For this review, take the finished solid that the model builds, in its own axes (mm). A direction names the side the tool comes from. Give positions to 0.01 mm unless a question says otherwise; leave off trailing zeros. Write each loop counter-clockwise with the first axis right and the second up, starting at its lowest first coordinate (ties: lowest second). Pieces come first, ordered by that corner, then holes.
1) We need section A-A on x = 0. Give the boundary of the cut face in (y, z).
2) We need section D-D on y = 101.5. Give the boundary of the cut face in (x, z), and give its area (3 significant figures).
3) For P1, Ø4, axis at x = -1, z = -91.5, coming from the +Y side; P2, Ø10, axis at x = 2.5, z = -95, coming from the -Y side; P3, Ø2.5, axis at x = -1, y = 93, coming from the -Z side; P4, Ø2, axis at x = -10, y = 76, coming from the +Z side, all flat-tipped, find the tip position at first contact; note any pin that passes through.
4) Wall thickness on line 1 along Y through (x, z) = (0, -77); line 2 along X through (y, z) = (92, -79.25); line 3 along Y through (x, z) = (-0.5, -97.5): over which ranges is each line inside the solid? List them lowest first.
5) We need section B-B on z = -80. Give the boundary of the cut face in (x, y), and give its area (3 significant figures).
6) Machinability: for faces 1 (the face through (-14, 92, -96)), 2 (the face through (-3.755, 103.923, -82.14)), 3 (the face through (-3.654, 94.071, -91.126)), which of the approach directions +Z, -Z, +X, -X, +Y, -Y give a long, thin tool a straight path to every point of the face, cutting with its end or side? Answer none if there is none.
7) Draft analysis for pull direction X (two halves, no side actions). For faces 4 (the face through (-13, 92, -92)), 5 (the face through (0, 96.2, -91)), 6 (the face through (3.654, 89.929, -91.126)), 7 (the face through (0.2, 117.5, -96.1)), state which applies: pulls with the +X half, pulls with the -X half, needs draft (parallel to the pull), parting line crosses it, or undercut.
8) We need section C-C on x = 8.75. Give the boundary of the cut face in (y, z).
from build123d import *

# Parameters (mm, degrees)
SKETCH151_W     = 65
SKETCH151_H     = 65
SKETCH151_W_2   = 53.065996
SKETCH151_H_2   = 28
POCKET099_DEPTH = 28.001
POCKET100_DEPTH = 18


with BuildPart() as part:
    # Sketch103 → Revolution002 (revolve)
    with BuildSketch(Plane.YZ):
        Polygon((2.75, 0), (12.5, 0), (12.5, -20), (25.5, -20), (25.5, -28), (2.75, -28), align=None)
    revolve(axis=Axis((0, 0, 0), (0, 0, 1)))

    # Sketch151 (on Face5 of Revolution002) → Pocket099 (cut, through all)
    with BuildSketch(Plane.YX.offset(28)):
        Rectangle(SKETCH151_W, SKETCH151_H)
        Rectangle(SKETCH151_W_2, SKETCH151_H_2, mode=Mode.SUBTRACT)
    extrude(amount=-POCKET099_DEPTH, mode=Mode.SUBTRACT)

    # Sketch142 (on Face5 of Revolution002) → Pocket100 (cut)
    with BuildSketch(Plane.YX.offset(28)):
        Polygon((4.2, 2.424871), (0, 4.849742), (-4.2, 2.424871), (-4.2, -2.424871), (0, -4.849742), (4.2, -2.424871), align=None)
    extrude(amount=-POCKET100_DEPTH, mode=Mode.SUBTRACT)


with BuildPart() as part_1:
    # Body022019 placement: moved
    add(part.part.moved(Location((0, 92, -72))))


solid = part_1.part
Results list:
1. outline: (66.5, -100) - (87.8, -100) - (87.8, -82) - (89.25, -82) - (89.25, -72) - (79.5, -72) - (79.5, -92) - (66.5, -92) - close; (94.75, -82) - (96.2, -82) - (96.2, -100) - (117.5, -100) - (117.5, -92) - (104.5, -92) - (104.5, -72) - (94.75, -72) - close
2. outline: (-14, -100) - (14, -100) - (14, -92) - (8.12, -92) - (8.12, -72) - (-8.12, -72) - (-8.12, -92) - (-14, -92) - close
2. area: 549 mm2
3. P1: stops at y = 117.5
3. P2: stops at y = 66.5
3. P3: passes through
3. P4: stops at z = -92
4. line 1: y = 79.5 to 89.25, 94.75 to 104.5
4. line 2: x = -12.5 to -2.75, 2.75 to 12.5
4. line 3: y = 66.5 to 87.8, 96.2 to 117.5
5. outline: circle Ø25 at (0, 92); hole circle Ø5.5 at (0, 92)
5. area: 467 mm2
6. face 1: +Z, -Z, -X, +Y, -Y
6. face 2: +Z
6. face 3: -Z
7. face 4: needs draft
7. face 5: undercut
7. face 6: undercut
7. face 7: parting line crosses it
8. outline: (68.05, -100) - (115.95, -100) - (115.95, -92) - (100.93, -92) - (100.93, -72) - (83.07, -72) - (83.07, -92) - (68.05, -92) - close
